Part print with two shaded views. Sizes in mm from the minimum x, y, z corner. A direction names the side the tool comes from. Coordinates: 2 decimals unless noted, no trailing zeros. Loops run counter-clockwise (first coordinate to the right, second up) from the corner with the lowest first, then second, coordinate; pieces in that order, holes last.
(1) Slice it at B-B (y = 20.25). Give the cut face in (x, z) (1 decimal).
(2) Flat gauge pins, fed straight in: P1, Ø1.4, axis at y = 22.5, z = 23.5, coming from the +X side (1 decimal); P2, Ø7, axis at y = 6.35, z = 36.576, coming from the +X side; P3, Ø1, axis at y = 22, z = 21.5, coming from the -X side; P4, Ø5, axis at x = 34.5, z = 27, coming from the -Y side. Where does each tip first touch, or does it go through?
(3) Slice it at C-C (x = 23.5). Give the cut face in (y, z) (1 decimal).
(4) Slice it at D-D (z = 15.5). Give the cut face in (x, y) (1 decimal).
(5) Wall check: L1, parallel to X at y = 13, z = 31 (1 decimal); L2, parallel to Y at x = 1, z = 6.35; L3, parallel to Y at x = 16, z = 11. Give the ranges that are in metal, low to high.
(6) Two-plate mould, pull along X, no slides. Class the marked faces 1, 2 and 3: pulls with the +X half, pulls with the -X half, needs draft (parallel to the pull), parting line crosses it, or undercut.
(7) Slice it at A-A (z = 6.35). Give the cut face in (x, y) (1 decimal).
(8) Tool access for the marked faces 4 and 5: list every direction of +Z, -Z, +X, -X, +Y, -Y with a clear straight run to the whole face (end or side of a thin tool).
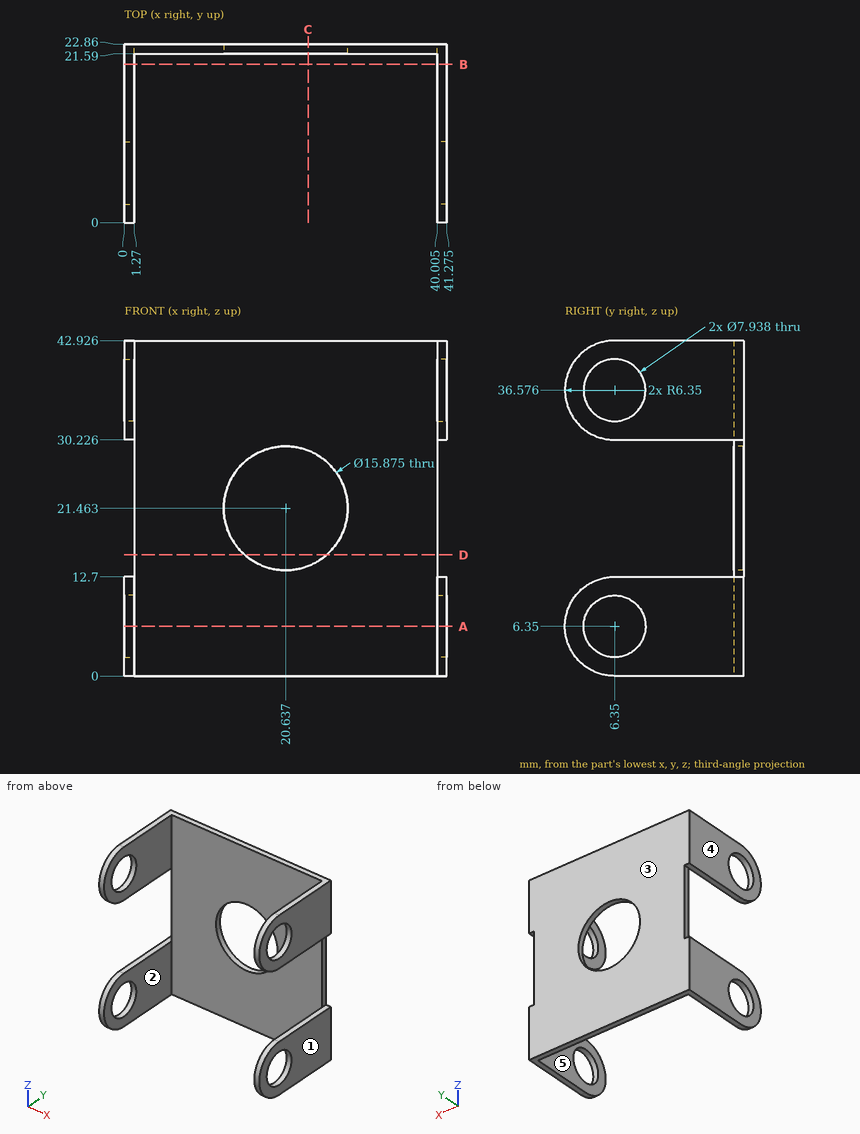
Response values:
1. outline: (0, 0) - (1.3, 0) - (1.3, 12.7) - (0, 12.7) - close; (0, 30.2) - (1.3, 30.2) - (1.3, 42.9) - (0, 42.9) - close; (40, 0) - (41.3, 0) - (41.3, 12.7) - (40, 12.7) - close; (40, 30.2) - (41.3, 30.2) - (41.3, 42.9) - (40, 42.9) - close
2. P1: stops at x = 40
2. P2: passes through
2. P3: stops at x = 1.27
2. P4: stops at y = 21.59
3. outline: (21.6, 0) - (22.9, 0) - (22.9, 14.1) - (21.6, 14.1) - close; (21.6, 28.9) - (22.9, 28.9) - (22.9, 42.9) - (21.6, 42.9) - close
4. outline: (1.3, 21.6) - (15.4, 21.6) - (15.4, 22.9) - (1.3, 22.9) - close; (25.9, 21.6) - (40, 21.6) - (40, 22.9) - (25.9, 22.9) - close
5. L1: x = 0 to 1.3, 40 to 41.3
5. L2: y = 0 to 2.38, 10.32 to 22.86
5. L3: y = 21.59 to 22.86
6. face 1: pulls with the +X half
6. face 2: undercut
6. face 3: needs draft
7. outline: (0, 0) - (1.3, 0) - (1.3, 2.4) - (0, 2.4) - close; (0, 10.3) - (1.3, 10.3) - (1.3, 21.6) - (40, 21.6) - (40, 10.3) - (41.3, 10.3) - (41.3, 22.9) - (0, 22.9) - close; (40, 0) - (41.3, 0) - (41.3, 2.4) - (40, 2.4) - close
8. face 4: +Z, -Z, -X, +Y, -Y
8. face 5: +Z, -Z, -Y
